from build123d import *

# Parameters (mm, degrees)
F0_W     = 647.7
F0_H     = 450.85
F0_W_2   = 622.3
F0_H_2   = 425.45
F1_DEPTH = 266.7
F2_W     = 692.15
F2_H     = 279.4
F3_DEPTH = 12.7
F4_W     = 622.3
F4_H     = 425.45
F5_DEPTH = 12.7


with BuildPart() as f1:
    # F0 (on Top) → F1 (new body)
    with BuildSketch(Plane.XY):
        with Locations((0.116292, 27.810883)):
            Rectangle(F0_W, F0_H)
        with Locations((0.116292, 27.810883)):
            Rectangle(F0_W_2, F0_H_2, mode=Mode.SUBTRACT)
    extrude(amount=F1_DEPTH)

    # F2 (on face) → F3 (join)
    with BuildSketch(Plane.XZ.offset(197.614117)):
        with Locations((0.116292, 133.35)):
            Rectangle(F2_W, F2_H)
    extrude(amount=F3_DEPTH)

    # F4 (on face) → F5 (join)
    with BuildSketch(Plane.XY.offset(266.7)):
        with Locations((0.116292, 27.810883)):
            Rectangle(F4_W, F4_H)
    extrude(amount=-F5_DEPTH)


solid = f1.part
Geometry: final body of the model. Coordinates: model frame, mm. A direction names the side the tool comes from. Round coordinates to 2 decimals unless told otherwise and drop trailing zeros. Loops run counter-clockwise (first coordinate to the right, second up) from the corner with the lowest first, then second, coordinate; pieces in that order, holes last.
Q1. Material intervals for L1, parallel to X at y = -138.5, z = 113.5; L2, parallel to Y at x = -50.5, z = 164; L3, parallel to Z at x = -75.5, y = 129, sorted ascending.
Q2. Pull-direction query (Y, two-part tool) for faces 1 (the flat face through (-313, 29, 0)), 2 (the flat face through (-4, -184.914, 125)), 3 (the flat face through (-5, -210.314, 135)); classes: released by +Y, released by -Y, zero draft, split by the parting line, or undercut.
Q3. Section A-A on z = 166. Return loops of the section in (x, y), plus the area to 3 significant figures.
Q4. Pin query (flat end, axial travel): P1, Ø4, axis at x = 198.5, y = 123.5, coming from the -Z side; P2, Ø12, axis at y = 71.5, z = 93, coming from the -X side; P3, Ø5, axis at x = -247.5, y = 115, coming from the +Z side. Return the tip coordinate at first contact, or that it passes through.
Q5. Access query for faces 4 (the flat face through (-323.734, 25, 131)), 5 (the flat face through (-4, 253.236, 131)), 6 (the flat face through (323.966, 25, 131)), 7 (the flat face through (311.266, 25, 125)), 8 (the flat face through (-4, 31, 266.7)). Directions: +Z, -Z, +X, -X, +Y, -Y. A direction counts if a zero-diameter tool reaches every point of the face in a straight line with its end or side. Return the directions, or none.
Q6. Section B-B on x = -275.5. Return loops of the section in (y, z), plus the area to 3 significant figures.
Q7. Section C-C on y = 80.5. Return loops of the section in (x, z), plus the area to 3 significant figures.
Evaluation:
1. L1: x = -323.73 to -311.03, 311.27 to 323.97
1. L2: y = -210.31 to -184.91, 240.54 to 253.24
1. L3: z = 254 to 266.7
2. face 1: zero draft
2. face 2: undercut
2. face 3: released by -Y
3. outline: (-345.96, -210.31) - (346.19, -210.31) - (346.19, -197.61) - (323.97, -197.61) - (323.97, 253.24) - (-323.73, 253.24) - (-323.73, -197.61) - (-345.96, -197.61) - close; hole (-311.03, -184.91) - (311.27, -184.91) - (311.27, 240.54) - (-311.03, 240.54) - close
3. area: 36,000 mm2
4. P1: stops at z = 254
4. P2: stops at x = -323.73
4. P3: stops at z = 266.7
5. face 4: +Z, -Z, -X, +Y
5. face 5: +Z, -Z, +X, -X, +Y
5. face 6: +Z, -Z, +X, +Y
5. face 7: -Z
5. face 8: +Z, +X, -X, +Y
6. outline: (-210.31, -6.35) - (-197.61, -6.35) - (-197.61, 0) - (-184.91, 0) - (-184.91, 254) - (240.54, 254) - (240.54, 0) - (253.24, 0) - (253.24, 266.7) - (-197.61, 266.7) - (-197.61, 273.05) - (-210.31, 273.05) - close
6. area: 15,700 mm2
7. outline: (-323.73, 0) - (-311.03, 0) - (-311.03, 254) - (311.27, 254) - (311.27, 0) - (323.97, 0) - (323.97, 266.7) - (-323.73, 266.7) - close
7. area: 14,700 mm2
